Verification items for the finished model (mm, model axes). Face numbers are marked on the shaded views. A direction names the side the tool comes from. Give positions to 0.01 mm unless a question says otherwise; leave off trailing zeros. Order: outer loops, then holes, each group sorted by start corner. A loop starts at its lowest first (then second) coordinate and runs counter-clockwise, first axis right, second up. Notation, with made-up numbers: (74, 6) - (118, 6) arc R37 cw to (118, 42) - close; hole circle Ø5 at (3, 3.25). An arc over 180 degrees is marked (long way). Answer as a JSON object with one key per item and string values.
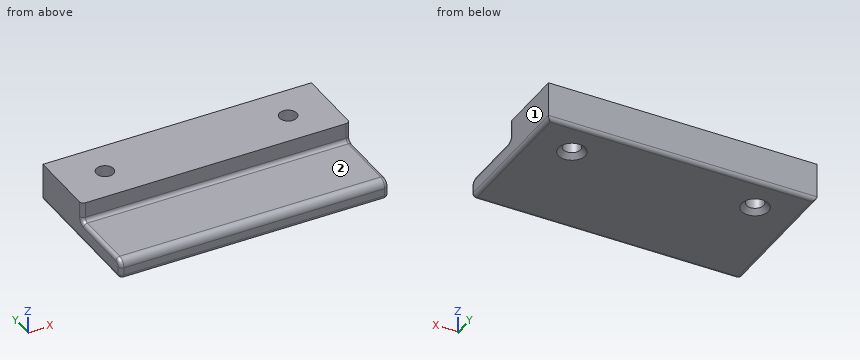
```python
from build123d import *

# Parameters (mm, degrees)
F0_W           = 70
F0_H           = 18.5
F1_DEPTH       = 10
F2_DEPTH       = 5
F3_R           = 2
F4_R           = 1
F5_D           = 4.5
F5_CSINK_D     = 7
F5_CSINK_ANGLE = 90


with BuildPart() as f1:
    # F0 (on Top) → F1 (new body)
    with BuildSketch(Plane.XY):
        with Locations((15.0051557424, 0)):
            Rectangle(F0_W, F0_H)
    extrude(amount=F1_DEPTH)

    # F0 (on Top) → F2 (join)
    with BuildSketch(Plane.XY):
        with Locations((15.0051557424, -18.5)):
            Rectangle(F0_W, F0_H)
    extrude(amount=F2_DEPTH)

    # F3
    f3_edges = [f1.edges().sort_by_distance(p)[0] for p in [
        (15.005156, -27.75, 5),
    ]]
    fillet(f3_edges, radius=F3_R)

    # F4
    f4_edges = [f1.edges().sort_by_distance(p)[0] for p in [
        (50.005156, -17.5, 5),
        (-19.994844, -17.5, 5),
        (50.005156, -9.25, 0),
        (15.005156, -27.75, 0),
        (-19.994844, -9.25, 0),
        (15.005156, 9.25, 0),
        (15.005156, -9.25, 5),
        (-19.994844, -27.164214, 4.414214),
        (-19.994844, -9.25, 7.5),
        (50.005156, -27.164214, 4.414214),
        (50.005156, -9.25, 7.5),
    ]]
    fillet(f4_edges, radius=F4_R)

    # F5 (through all)
    with Locations(Plane(origin=(0, 0, 0), x_dir=(1, 0, 0), z_dir=(0, 0, -1))):
        with Locations((-8.8698442576, 0), (38.8801557424, 0)):
            CounterSinkHole(F5_D / 2, F5_CSINK_D / 2, counter_sink_angle=F5_CSINK_ANGLE)


solid = f1.part
```
(1) Material ranges on line 1 along X through (y, z) = (0.5, 6.75); line 2 along Z through (x, y) = (36, -13.5); line 3 along Y through (x, z) = (-7.5, 8), recorded low to high. Write a range as [from, to].
Computed values:
{"line 1": "x = [-19.99, -11.06], [-6.68, 36.69], [41.07, 50.01]", "line 2": "z = [0, 5]", "line 3": "y = [-9.25, -1.78], [1.78, 9.25]"}
(2) Section check A-A (y = 0). Record the cut outline in (x, z).
Computed values:
{"outline": "(-19.99, 1) arc R1 ccw to (-18.99, 0) - (-12.37, 0) - (-11.12, 1.25) - (-11.12, 10) - (-19.99, 10) - close; (-6.62, 1.25) - (-5.37, 0) - (35.38, 0) - (36.63, 1.25) - (36.63, 10) - (-6.62, 10) - close; (41.13, 1.25) - (42.38, 0) - (49.01, 0) arc R1 ccw to (50.01, 1) - (50.01, 10) - (41.13, 10) - close"}
(3) Gauge pin test, flat ends, axial feed: pin 1 Ø12.5 at (x, y) = (31.5, -16.5) entering from +Z; pin 2 Ø4.5 at (x, z) = (19, 7) entering from -Y; pin 3 Ø2 at (y, z) = (-11.5, 8) entering from +X; pin 4 Ø5 at (x, z) = (16, 7) entering from -Y. Record the tip position at first contact, or that the pin passes through.
Computed values:
{"pin 1": "stops at z = 5", "pin 2": "stops at y = -26.72", "pin 3": "passes through", "pin 4": "stops at y = -27.07"}
(4) Section check C-C (z = 6.75). Record the cut outline in (x, y), then the cut area to 3 significant figures.
Computed values:
{"outline": "(-19.99, -8.25) arc R1 ccw to (-18.99, -9.25) - (49.01, -9.25) arc R1 ccw to (50.01, -8.25) - (50.01, 9.25) - (-19.99, 9.25) - close; hole circle Ø4.5 at (-8.87, 0); hole circle Ø4.5 at (38.88, 0)", "area": "1,260 mm²"}
(5) Section check D-D (y = -11). Record the cut outline in (x, z).
Computed values:
{"outline": "(-19.99, 1) arc R1 ccw to (-18.99, 0) - (49.01, 0) arc R1 ccw to (50.01, 1) - (50.01, 4) arc R1 ccw to (49.01, 5) - (-18.99, 5) arc R1 ccw to (-19.99, 4) - close"}
(6) Section check B-B (x = -14.5). Record the cut outline in (y, z).
Computed values:
{"outline": "(-27.75, 1) arc R1 ccw to (-26.75, 0) - (8.25, 0) arc R1 ccw to (9.25, 1) - (9.25, 10) - (-9.25, 10) - (-9.25, 6) arc R1 cw to (-10.25, 5) - (-25.75, 5) arc R2 ccw to (-27.75, 3) - close"}
(7) Access from +Z, -Z, +X, -X, +Y, -Y to the whole of each face (thin tool, end or side, straight path). Record for the marked faces 1 and 2.
Computed values:
{"face 1": "+Z, -Z, +X, +Y, -Y", "face 2": "+Z, +X, -X, -Y"}
